```python
from build123d import *

# Parameters (mm, degrees)
MASTER_CYLINDER_BODY_DEPTH             = 77.978
MASTER_CYLINDER_BODY_DEPTH_BACK        = 4.572
SKETCH1_R                              = 18.796
MASTER_START                           = -7.874
MASTER_CYLINDER_MOUNTS_OUTLINE_R       = 5.08
MASTER_CYLINDER_MOUNTS_OUTLINE_R_2     = 18.796
MASTER_CYLINDER_MOUNTS_DEPTH           = 7.874
SKETCH3_R                              = 11.1125
SKETCH3_R_2                            = 8.73125
RESERVOIR_MOUNT_DEPTH                  = 15.875
RESERVOIR_MOUNT_DIRECTION_2_REACH      = 100.39
RESERVOIR_MOUNT_DIRECTION_2_END_RADIUS = 18.796
SKETCH5_R                              = 8.89
MASTER_CYLINDER_OUTLET_DEPTH           = 7.366
SKETCH6_R                              = 3.96875
PUSHROD_DEPTH                          = 108.712
SKETCH7_R                              = 20.32
RUBBER_COVER_DEPTH                     = 44.45


# Read off the part's stored shape, not the designer's step: Master Cylinder Mounts
with BuildPart() as part:
    # Sketch1 → Master Cylinder Body (new, two sides: drawn at the far end of the back side and taken through both)
    with BuildSketch(Plane.XY.offset(-MASTER_CYLINDER_BODY_DEPTH_BACK)):
        Circle(SKETCH1_R)
    extrude(amount=MASTER_CYLINDER_BODY_DEPTH + MASTER_CYLINDER_BODY_DEPTH_BACK)

    # Master Cylinder Mounts outline → Master Cylinder Mounts (add)
    with BuildSketch(Plane(origin=(0, 0, 0), x_dir=(-1, 0, 0), z_dir=(0, 0, -1)).offset(MASTER_START)):
        with BuildLine():
            ThreePointArc((-8.312226974, -33.226075976), (0, -38.1), (8.312226974, -33.226075976))
            Line((8.312226974, -33.226075976), (19.05, -14.035934373))
            Line((19.05, -14.035934373), (19.05, 14.035934373))
            Line((19.05, 14.035934373), (8.312226974, 33.226075976))
            ThreePointArc((8.312226974, 33.226075976), (0, 38.1), (-8.312226974, 33.226075976))
            Line((-8.312226974, 33.226075976), (-19.05, 14.035934373))
            Line((-19.05, 14.035934373), (-19.05, -14.035934373))
            Line((-19.05, -14.035934373), (-8.312226974, -33.226075976))
        make_face()
        with Locations((0, -28.575)):
            Circle(MASTER_CYLINDER_MOUNTS_OUTLINE_R, mode=Mode.SUBTRACT)
        Circle(MASTER_CYLINDER_MOUNTS_OUTLINE_R_2, mode=Mode.SUBTRACT)
        with Locations((0, 28.575)):
            Circle(MASTER_CYLINDER_MOUNTS_OUTLINE_R, mode=Mode.SUBTRACT)
    extrude(amount=MASTER_CYLINDER_MOUNTS_DEPTH)

    # Sketch3 → Reservoir Mount (add)
    with BuildSketch(Plane(origin=(0, 18.796, 0), x_dir=(1, 0, 0), z_dir=(0, 1, 0))):
        with Locations(Location((0, -37.084, 0), (0, 0, 270))):
            Circle(SKETCH3_R)
        with Locations(Location((0, -37.084, 0), (0, 0, 90))):
            Circle(SKETCH3_R_2, mode=Mode.SUBTRACT)
    extrude(amount=RESERVOIR_MOUNT_DEPTH)

    # Reservoir Mount direction 2: up to this cylinder (the profile starts outside it)
    reservoir_mount_direction_2_end = Plane(origin=(0, 0, 26.285809), z_dir=(0, 0, 1)) * Cylinder(RESERVOIR_MOUNT_DIRECTION_2_END_RADIUS, 239.372, mode=Mode.PRIVATE)
    # Sketch3 → Reservoir Mount direction 2 (add, up to the surface)
    with BuildSketch(Plane(origin=(0, 18.796, 0), x_dir=(1, 0, 0), z_dir=(0, 1, 0)), mode=Mode.PRIVATE) as reservoir_mount_direction_2_sk1:
        with Locations(Location((0, -37.084, 0), (0, 0, 270))):
            Circle(SKETCH3_R)
        with Locations(Location((0, -37.084, 0), (0, 0, 90))):
            Circle(SKETCH3_R_2, mode=Mode.SUBTRACT)
    reservoir_mount_direction_2_tool1 = extrude(reservoir_mount_direction_2_sk1.sketch, amount=-RESERVOIR_MOUNT_DIRECTION_2_REACH, mode=Mode.PRIVATE) - reservoir_mount_direction_2_end
    add(reservoir_mount_direction_2_tool1.solids().sort_by_distance((0, 18.796, 26.285809))[0])
    add(reservoir_mount_direction_2_tool1.solids().sort_by_distance((0, 18.796, 26.285809))[1])

    # Sketch5 → Master Cylinder Outlet (add)
    with BuildSketch(Plane.XY.offset(77.978)):
        with Locations(Location((0, 9.906, 0), (0, 0, 90))):
            Circle(SKETCH5_R)
    extrude(amount=MASTER_CYLINDER_OUTLET_DEPTH)

    # Sketch6 → Pushrod (add)
    with BuildSketch(Plane(origin=(0, 0, -4.572), x_dir=(-1, 0, 0), z_dir=(0, 0, -1))):
        with Locations(Location((0, 0, 0), (0, 0, 180))):
            Circle(SKETCH6_R)
    extrude(amount=PUSHROD_DEPTH)

    # Sketch7 → Rubber Cover (add)
    with BuildSketch(Plane(origin=(0, 0, -4.572), x_dir=(-1, 0, 0), z_dir=(0, 0, -1))):
        Circle(SKETCH7_R)
    extrude(amount=RUBBER_COVER_DEPTH)


solid = part.part
```
Work out the finished part from the listing and answer in its coordinate system (mm). A direction names the side the tool comes from. Give positions to 0.01 mm unless a question says otherwise; leave off trailing zeros. Write each loop counter-clockwise with the first axis right and the second up, starting at its lowest first coordinate (ties: lowest second). Pieces come first, ordered by that corner, then holes. Notation, with made-up numbers: (86.5, 73.5) -> (115.5, 73.5) arc R22 ccw to (115.5, 93.5) -> close; hole circle Ø10 at (43.5, 37). An arc over 180 degrees is marked (long way). Write each question's results on one line, items separated by ' | '.
1. Find section B-B on z = 50.5. Determine the outline of the cut face in (x, y).
Data:
outline: circle Ø37.59 at (0, 0)
2. Each of these flat-tipped pins is pushed along its axis until it touches: pin 1 Ø6.5 at (x, z) = (-3.5, 34.5) entering from +Y; pin 2 Ø6.5 at (y, z) = (-6, 3) entering from +X; pin 3 Ø1 at (x, y) = (-8.5, -18) entering from +Z. Where does it stop, or does it pass through?
Data:
pin 1: y = 18.79 | pin 2: x = 19.05 | pin 3: z = 7.87
3. Determine the mould class of faces 1 (the flat face through (-13, 14, 7.874)), 2 (the cylindrical face through (2.645, 20.147, -26.486)), 3 (the flat face through (0, 10, 85.344)), 4 (the cylindrical face through (-2.447, 18.636, -2.318)) for opening direction Z: +Z half, -Z half, draft (parallel to the pull), parting line (faces both ways), or undercut.
Data:
face 1: undercut | face 2: draft | face 3: +Z half | face 4: undercut
4. Find section A-A on y = -26.5. Determine the outline of the cut face in (x, z).
Data:
outline: (-12.08, 0) -> (-4.64, 0) -> (-4.64, 7.87) -> (-12.08, 7.87) -> close; (4.64, 0) -> (12.08, 0) -> (12.08, 7.87) -> (4.64, 7.87) -> close
5. Straight lines are drawn through the part: L1, parallel to Y at x = 0, z = 3.5 (3 decimals); L2, parallel to Z at x = -9, y = -17; L3, parallel to Z at x = -4, y = 12.5. For each, find the intervals that lie inside material, in ascending order.
Data:
L1: -38.1 to -33.655, -23.495 to 23.495, 33.655 to 38.1 | L2: -49.02 to -4.57, 0 to 7.87 | L3: -49.02 to 85.34
6. Find section C-C on y = -16. Determine the outline of the cut face in (x, z), and give its area (3 significant figures).
Data:
outline: (-17.95, 0) -> (-9.86, 0) -> (-9.86, -4.57) -> (-12.53, -4.57) -> (-12.53, -49.02) -> (12.53, -49.02) -> (12.53, -4.57) -> (9.86, -4.57) -> (9.86, 0) -> (17.95, 0) -> (17.95, 7.87) -> (9.86, 7.87) -> (9.86, 77.98) -> (-9.86, 77.98) -> (-9.86, 7.87) -> (-17.95, 7.87) -> close | area: 2,870 mm^2
7. Find section D-D on x = -16. Determine the outline of the cut face in (y, z), and give its area (3 significant figures).
Data:
outline: (-19.49, 0) -> (-9.86, 0) -> (-9.86, -4.57) -> (-12.53, -4.57) -> (-12.53, -49.02) -> (12.53, -49.02) -> (12.53, -4.57) -> (9.86, -4.57) -> (9.86, 0) -> (19.49, 0) -> (19.49, 7.87) -> (9.86, 7.87) -> (9.86, 77.98) -> (-9.86, 77.98) -> (-9.86, 7.87) -> (-19.49, 7.87) -> close | area: 2,890 mm^2
8. A tool of negligible diameter and unlimited length cuts with its end or side. For faces 5 (the flat face through (19.05, 0, 4)), 6 (the flat face through (-6, 34.671, 30)), 7 (the flat face through (13.606, 23.765, 3.992)), 8 (the flat face through (-13.756, 23.497, 3.992)), from which of +Z, -Z, +X, -X, +Y, -Y can it reach the whole face along a straight path? Write none if from no direction.
Data:
face 5: +Z, +X, +Y, -Y | face 6: +Z, +X, -X, +Y | face 7: -Z, +X, +Y | face 8: -Z, -X, +Y
